Autodesk Inventor part; units mm, degrees
ref_plane "YZ Plane" through (0, 0, 0) normal (1, 0, 0) x (0, 1, 0)
ref_plane "XZ Plane" through (0, 0, 0) normal (0, 1, 0) x (-1, 0, 0)
ref_plane "XY Plane" through (0, 0, 0) normal (0, 0, 1) x (1, 0, 0)
sketch "Sketch1" plane through (0, 0, 0) normal (0, 0, 1) x (1, 0, 0)
  circle A0 centre (0, 0) radius 2.5
  dimension "d0" = 5
extrude "Extrusion1" add sketch "Sketch1" along normal blind 320
sketch "Sketch2" plane through (0, 0, 320) normal (0, 0, 1) x (1, 0, 0)
  circle A0 centre (0, 0) radius 2.5
  circle A1 centre (0, 0) radius 1
  dimension "d3" = 2
extrude "Extrusion2" add sketch "Sketch2" along normal blind 3 contours A1
sketch "Sketch3" plane through (0, 0, 0) normal (0, 0, -1) x (-1, 0, 0)
  circle A0 centre (0, 0) radius 1
  dimension "d6" = 2
extrude "Extrusion3" add sketch "Sketch3" along normal blind 3
properties part number "Bone-32cm"
Model file for the job. Use its own axes, mm. A direction names the side the tool comes from. Give positions to 0.01 mm unless a question says otherwise; leave off trailing zeros. Loops run counter-clockwise (first coordinate to the right, second up) from the corner with the lowest first, then second, coordinate; pieces in that order, holes last.
1) Tool access for faces 1 (the flat face through (1, -1, 0)), 2 (the cylindrical face through (-0.54, 2.44, 157.76)), 3 (the flat face through (1, -1, 320)): list every direction of +Z, -Z, +X, -X, +Y, -Y with a clear straight run to the whole face (end or side of a thin tool).
2) Saw through at A-A (z = 24). Write the cut outline in (x, y), plus the area to 3 significant figures.
3) Wall check: line 1 (Z direction, x = 2.1, y = 1.15); line 2 (X direction, y = 0.45, z = 54); line 3 (Y direction, x = -2.3, z = 305.5). Give the ranges that are in metal, low to high.
4) Flat gauge pin, fed straight in: pin 1 Ø1.5 at (y, z) = (-1.5, 164.5) entering from +X. Where does the tip first touch, or does it go through?
Answer block:
1. face 1: -Z
1. face 2: +Z, -Z
1. face 3: +Z
2. outline: circle Ø5 at (0, 0)
2. area: 19.6 mm2
3. line 1: z = 0 to 320
3. line 2: x = -2.46 to 2.46
3. line 3: y = -0.98 to 0.98
4. pin 1: stops at x = 2.38
